Here's how the part is built. I have some questions about the finished solid (model axes, mm). Coordinates: 2 decimals unless noted, no trailing zeros. Write each loop counter-clockwise with the first axis right and the second up, starting at its lowest first coordinate (ties: lowest second). Pieces come first, ordered by that corner, then holes.
Item 1: I want a section at C-C (x = 63.5). Please give me the cut outline in (y, z), and give its area (3 significant figures).
Item 2: Please list where these lines run through material, in increasing order: line 1 (Y direction, x = 35, z = 0.55); line 2 (X direction, y = 12.5, z = 0.5); line 3 (X direction, y = -38, z = 0.65).
Item 3: I want a section at D-D (z = 0.45). Count the separate pieces of the cut face and the enclosed holes in it, and give its area (3 significant figures).
Item 4: If we mould it in two halves opening along X, with no side actions, what happens to faces 1 (the face through (15.59, -76.72, 0.39)), 2 (the face through (56, -33, 0)), 3 (the face through (25.24, -45.63, 0.4))? For each: pulls with the +X half, pulls with the -X half, needs draft (parallel to the pull), parting line crosses it, or undercut.
Item 5: I want a section at B-B (y = 28). Please give me the cut outline in (x, z), and give its area (3 significant figures).
Item 6: I'm going to push a flat-ended pin straight in: P1, Ø7.5, axis at x = 65.92, y = -50.87, coming from the +Z side. Where does the tip first touch, or does it pass through?
Item 7: I want a section at A-A (x = 48.5). Please give me the cut outline in (y, z), and give its area (3 significant figures).
Autodesk Inventor part; units mm, degrees
ref_plane "YZ Plane" through (0, 0, 0) normal (1, 0, 0) x (0, 1, 0)
ref_plane "XZ Plane" through (0, 0, 0) normal (0, 1, 0) x (-1, 0, 0)
ref_plane "XY Plane" through (0, 0, 0) normal (0, 0, 1) x (1, 0, 0)
sketch "Sketch1" plane through (0, 0, 0) normal (0, 0, 1) x (1, 0, 0)
  line L0 (11.7695, 33.9618) -> (11.7695, -67.6382)
  line L1 (100.6695, 33.9618) -> (100.6695, -67.6382)
  line L2 (18.1195, 40.3118) -> (94.3195, 40.3118)
  line L3 (24.4695, -80.3382) -> (87.9695, -80.3382)
  arc A0 (11.7695, -67.6382) -> (24.4695, -80.3382) centre (24.4695, -67.6382) ccw
  arc A1 (87.9695, -80.3382) -> (100.6695, -67.6382) centre (87.9695, -67.6382) ccw
  arc A2 (100.6695, 33.9618) -> (94.3195, 40.3118) centre (94.3195, 33.9618) ccw
  arc A3 (18.1195, 40.3118) -> (11.7695, 33.9618) centre (18.1195, 33.9618) ccw
  point P0 (0, 0)
  dimension "d0" = 12.7
  dimension "d1" = 6.35
  dimension "d2" = 120.65
  dimension "d3" = 88.9
extrude "Extrusion1" add sketch "Sketch1" along normal blind 0.7937
sketch "Sketch2" plane through (0, 0, 0.7937) normal (0, 0, 1) x (1, 0, 0)
  line L0 (11.7695, -67.6382) -> (11.7695, 33.9618)
  line L1 (100.6695, 33.9618) -> (100.6695, -67.6382)
  line L2 (18.1195, 40.3118) -> (94.3195, 40.3118)
  line L3 (19.7795, 32.2228) -> (92.6595, 32.2228)
  line L4 (92.6595, 32.2228) -> (92.6595, -23.1372)
  line L5 (92.6595, -23.1372) -> (19.7795, -23.1372)
  line L6 (19.7795, -23.1372) -> (19.7795, 32.2228)
  line L7 (87.9695, -80.3382) -> (24.4695, -80.3382)
  point P0 (0, 0)
  dimension "d7" = 8.089
  dimension "d22" = 72.88
  dimension "d23" = 8.01
  dimension "d24" = 8.01
  dimension "d25" = 55.36
  dimension "d70" = 80.89
  dimension "d71" = 57.201
  dimension "d72" = 112.561
extrude "Extrusion2" cut sketch "Sketch2" against normal through all
sketch "Sketch5" plane through (0, 0, 0.7937) normal (0, 0, 1) x (1, 0, 0)
  circle A0 centre (34.6295, -46.0482) radius 9.398
  circle A1 centre (82.6355, -41.2222) radius 4.572
  circle A2 centre (65.9178, -50.8742) radius 4.572
  line L0 (87.9695, -80.3382) -> (24.4695, -80.3382)
  line L1 (11.7695, -67.6382) -> (11.7695, 33.9618)
  line L2 (100.6695, 33.9618) -> (100.6695, -67.6382)
  line L3 (100.6695, -46.0482) -> (11.7695, -46.0482) construction
  line L4 (65.9178, -50.8742) -> (74.2766, -46.0482) construction
  line L5 (82.6355, -41.2222) -> (74.2766, -46.0482) construction
  line L6 (25.2315, -36.6502) -> (87.2075, -36.6502) construction
  line L7 (87.2075, -36.6502) -> (87.2075, -55.4462) construction
  line L8 (87.2075, -55.4462) -> (25.2315, -55.4462) construction
  line L9 (25.2315, -55.4462) -> (25.2315, -36.6502) construction
  point P0 (0, 0)
  dimension "d26" = 18.796
  dimension "d27" = 9.144
  dimension "d35" = 34.29
  dimension "d40" = 30
  dimension "d41" = 13.462
  dimension "d42" = 13.462
  dimension "d54" = 66.04
  dimension "d55" = 34.7518
  dimension "d56" = 18.034
  dimension "d57" = 29.464
  dimension "d58" = 39.116
extrude "Extrusion5" cut sketch "Sketch5" against normal through all
sketch "Sketch6" plane through (0, 0, 0.7937) normal (0, 0, 1) x (1, 0, 0)
  line L0 (52.111, -71.628) -> (60.3281, -71.628)
  arc A0 (52.111, -71.628) -> (49.1232, -73.533) centre (50.5369, -72.4548) ccw
  arc A1 (49.1232, -73.533) -> (52.111, -75.438) centre (50.5369, -74.6113) ccw
  line L1 (52.111, -75.438) -> (60.3281, -75.438)
  arc A2 (63.3159, -73.533) -> (60.3281, -71.628) centre (61.9022, -72.4548) ccw
  arc A3 (60.3281, -75.438) -> (63.3159, -73.533) centre (61.9022, -74.6113) ccw
  line L2 (11.7695, -67.6382) -> (11.7695, 33.9618)
  point P0 (0, 0)
  dimension "d43" = 3.81
  dimension "d44" = 1.778
  dimension "d45" = 8.2171
  dimension "d51" = 40.3415
  dimension "d52" = 2.1565
extrude "Extrusion6" [suppressed]
sketch "Sketch7" plane through (0, 0, 0.7937) normal (0, 0, 1) x (1, 0, 0)
  line L0 (11.7695, -67.6382) -> (11.7695, 33.9618)
  line L1 (87.9695, -80.3382) -> (24.4695, -80.3382)
  line L2 (100.6695, 33.9618) -> (100.6695, -67.6382)
  line L3 (18.1195, 40.3118) -> (94.3195, 40.3118)
  circle A0 centre (37.1695, 37.1876) radius 1.27
  circle A1 centre (75.2695, 37.1876) radius 1.27
  circle A2 centre (97.5453, 21.2618) radius 1.27
  circle A3 centre (97.5453, -16.8382) radius 1.27
  circle A4 centre (75.2695, -77.214) radius 1.27
  circle A5 centre (37.1695, -77.214) radius 1.27
  circle A6 centre (14.8937, 21.2618) radius 1.27
  circle A7 centre (14.8937, -16.8382) radius 1.27
  point P0 (0, 0)
  dimension "d59" = 2.54
  dimension "d60" = 3.1242
  dimension "d61" = 3.1242
  dimension "d62" = 3.1242
  dimension "d63" = 3.1242
  dimension "d64" = 25.4
  dimension "d65" = 19.05
  dimension "d66" = 38.1
  dimension "d67" = 38.1
extrude "Extrusion7" cut sketch "Sketch7" against normal through all
equation "\"d23\" = d24"
equation "\"d42\" = d41"
properties part number "lcd_spacer"
Answer:
1. outline: (-80.34, 0) - (-54.75, 0) - (-54.75, 0.79) - (-80.34, 0.79) - close; (-46.99, 0) - (-23.14, 0) - (-23.14, 0.79) - (-46.99, 0.79) - close; (32.22, 0) - (40.31, 0) - (40.31, 0.79) - (32.22, 0.79) - close
1. area: 45.7 mm2
2. line 1: y = -80.34 to -55.44, -36.66 to -23.14, 32.22 to 40.31
2. line 2: x = 11.77 to 19.78, 92.66 to 100.67
2. line 3: x = 11.77 to 29.78, 39.48 to 79.39, 85.88 to 100.67
3. separate pieces: 1
3. enclosed holes: 12
3. area: 6,160 mm2
4. face 1: pulls with the -X half
4. face 2: needs draft
4. face 3: undercut
5. outline: (11.77, 0) - (19.78, 0) - (19.78, 0.79) - (11.77, 0.79) - close; (92.66, 0) - (100.67, 0) - (100.67, 0.79) - (92.66, 0.79) - close
5. area: 12.7 mm2
6. P1: passes through
7. outline: (-80.34, 0) - (-23.14, 0) - (-23.14, 0.79) - (-80.34, 0.79) - close; (32.22, 0) - (40.31, 0) - (40.31, 0.79) - (32.22, 0.79) - close
7. area: 51.8 mm2
